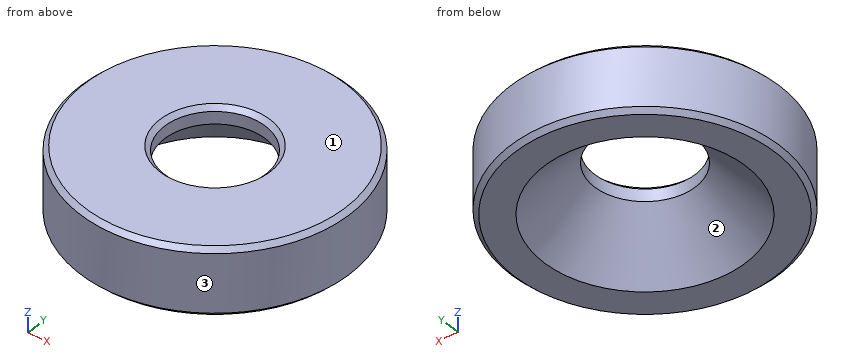
Autodesk Inventor part; units mm, degrees
ref_plane "YZ Plane" through (0, 0, 0) normal (1, 0, 0) x (0, 1, 0)
ref_plane "XZ Plane" through (0, 0, 0) normal (0, 1, 0) x (-1, 0, 0)
ref_plane "XY Plane" through (0, 0, 0) normal (0, 0, 1) x (1, 0, 0)
sketch "Sketch4" plane through (0, 0, 0) normal (0, 0, 1) x (1, 0, 0)
  circle A0 centre (0, 0) radius 6
  circle A1 centre (0, 0) radius 2.25
  dimension "d0" = 4.5
  dimension "d1" = 12
extrude "Extrusion1" add sketch "Sketch4" against normal blind 3
sketch "Sketch6" plane through (0, 0, 0) normal (0, 1, 0) x (-1, 0, 0)
  line L0 (0, -3) -> (4.5, -3)
  line L1 (4.5, -3) -> (0, 1.5)
  line L2 (0, -3) -> (0, 1.5)
  point P0 (0, 0)
  dimension "d12" = 45
  dimension "d13" = 9
  dimension "d15" = 3
revolve "Revolution1" cut sketch "Sketch6" angle 360 about axis through (0, 0, -3) along (0, 0, 1)
chamfer "Chamfer1" distance 0.2 angle 45 3 edges at (-6, 0, -3) (-6, 0, 0) (-2.25, 0, 0)
chamfer "Chamfer2" [suppressed]
equation "\"d0\" = Inside_Diameter"
equation "\"d1\" = Outside_Diameter"
equation "\"d2\" = Thickness"
equation "\"d13\" = 2 * Inside_Diameter"
equation "\"d4\" = Chamfer"
equation "\"d16\" = Chamfer"
equation "\"Outside_Diameter\" = 12"
equation "\"Inside_Diameter\" = 4.5"
equation "\"Thickness\" = 3"
equation "\"Chamfer\" = 0.2"
properties part number "FWSRS-D12-V4.5-E2.5-T3" material "Stainless Steel"
Model file for the job. Use its own axes, mm. Face numbers are marked on the shaded views. Give positions to 0.01 mm unless a question says otherwise; leave off trailing zeros. Order: outer loops, then holes, each group sorted by start corner. A loop starts at its lowest first (then second) coordinate and runs counter-clockwise, first axis right, second up. Notation, with made-up numbers: (0, -23.5) -> (36, -23.5) arc R12 ccw to (36, -15.5) -> close; hole circle Ø11 at (-1.5, 70). An arc over 180 degrees is marked (long way). Use CSV: the item, a comma, the result in double quotes.
1. Band-saw the part on A-A, the plane y = 0. Give the cut face in (x, z).
Outcome:
outline,"(-6, -2.8) -> (-5.8, -3) -> (-4.5, -3) -> (-2.25, -0.75) -> (-2.25, -0.2) -> (-2.45, 0) -> (-5.8, 0) -> (-6, -0.2) -> close; (2.25, -0.75) -> (4.5, -3) -> (5.8, -3) -> (6, -2.8) -> (6, -0.2) -> (5.8, 0) -> (2.45, 0) -> (2.25, -0.2) -> close"
2. Mould opens along X. For the marked faces 1, 2 and 3 say: +X half, -X half, draft (parallel to the pull), parting line (faces both ways), or undercut.
Outcome:
face 1,"draft"
face 2,"undercut"
face 3,"parting line"
3. Band-saw the part on D-D, the plane z = -1.1. Give the cut face in (x, y).
Outcome:
outline,"circle Ø12 at (0, 0); hole circle Ø5.2 at (0, 0)"
4. Drop flat-ended pins along their axis: pin 1 (1.5 mm diameter, centred on x = -3, y = 0.5, fed in from -Z); pin 2 (1 mm diameter, centred on x = -2.5, y = -2.5, fed in from -Z). Give the stop position or say it passes through.
Outcome:
pin 1,"z = -2.29"
pin 2,"z = -2.54"
5. Band-saw the part on C-C, the plane z = -2.55. Give the cut face in (x, y).
Outcome:
outline,"circle Ø12 at (0, 0); hole circle Ø8.1 at (0, 0)"
6. Drill centre lines: line 1 along Y through (x, z) = (0, -0.25); line 2 along X through (y, z) = (2.75, -2.75); line 3 along X through (y, z) = (0.75, -2.6). Where is each one in solid material? Low to high. Write a range as from..to.
Outcome:
line 1,"-6..-2.25, 2.25..6"
line 2,"-5.33..-3.24, 3.24..5.33"
line 3,"-5.95..-4.03, 4.03..5.95"
